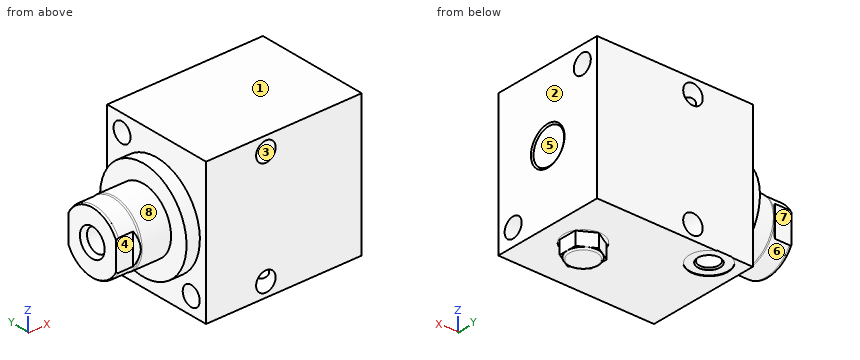
from build123d import *

# Parameters (mm, degrees)
SKETCH1_W            = 63.5
SKETCH1_H            = 50.8
EXTRUDE1_DEPTH       = 69.723
LPATTERN1_COUNT      = 2
LPATTERN1_PITCH      = 41.148
LPATTERN1_COUNT_DIR2 = 2
LPATTERN1_PITCH_DIR2 = 17.4498
SKETCH5_R            = 22.225
EXTRUDE2_DEPTH       = 5.969
SKETCH6_W            = 14.2748
SKETCH6_H            = 22.86
CUT_EXTRUDE4_DEPTH   = 30.48
HOLE1_D              = 8.738
HOLE1_DEPTH          = 69.723
HOLE2_D              = 8.738
HOLE2_DEPTH          = 50.8
EXTRUDE3_DEPTH       = 6.78
SKETCH21_R           = 7.874
EXTRUDE4_DEPTH       = 2.54


with BuildPart() as part:
    # Sketch1 → Extrude1 (new body)
    with BuildSketch(Plane(origin=(0, 0, 0), x_dir=(0, 0, -1), z_dir=(1, 0, 0))):
        Rectangle(SKETCH1_W, SKETCH1_H)
    extrude(amount=EXTRUDE1_DEPTH)

    # S2D0002 → Cut-Revolve1 (revolve, cut)
    with BuildSketch(Plane(origin=(0, 17.4498, 0), x_dir=(-1, 0, 0), z_dir=(0, 1, 0)), mode=Mode.PRIVATE) as cut_revolve1_sk:
        Polygon((-17.7165, -31.496), (-21.336, -31.496), (-21.336, -31.75), (-12.7, -31.75), (-12.7, -18.034), (-17.1196, -18.034), (-17.1196, -30.8737), (-17.7165, -31.4706), align=None)
    cut_revolve1 = revolve(cut_revolve1_sk.sketch.rotate(Axis((12.7, 17.4498, -19.13842003), (0, 0, 1)), 180), axis=Axis((12.7, 17.4498, -19.13842003), (0, 0, 1)), mode=Mode.SUBTRACT)  # turned: the seam where the file's is

    # LPattern1: Cut-Revolve1 2 × 2, 2 skipped
    with Locations(*[(i * LPATTERN1_PITCH, -j * LPATTERN1_PITCH_DIR2, 0) for i in range(LPATTERN1_COUNT) for j in range(LPATTERN1_COUNT_DIR2) if (i, j) not in ((0, 0), (0, 1), (1, 0))]):
        add(cut_revolve1, mode=Mode.SUBTRACT)

    # Sketch5 → Extrude2 (add)
    with BuildSketch(Plane.ZY):
        Circle(SKETCH5_R)
    extrude(amount=EXTRUDE2_DEPTH)

    # Sketch6 → Revolve1 (revolve)
    with BuildSketch(Plane(origin=(0, 0, 0), x_dir=(0, 0, 1), z_dir=(0, -1, 0)), mode=Mode.PRIVATE) as revolve1_sk:
        with Locations((-7.1374, 17.399)):
            Rectangle(SKETCH6_W, SKETCH6_H)
    revolve(revolve1_sk.sketch.rotate(Axis((5.754582971, 0, 0), (-1, 0, 0)), 180), axis=Axis((5.754582971, 0, 0), (-1, 0, 0)))  # turned: the seam where the file's is

    # S2D0001 → Cut-Revolve4 (revolve, cut)
    with BuildSketch(Plane(origin=(-18.511260017, 3.2639, 0), x_dir=(0, 1, 0), z_dir=(0, 0, 1)), mode=Mode.PRIVATE) as cut_revolve4_sk:
        Polygon((1.8669, 8.206023638), (1.8669, -6.522460017), (-3.2639, -6.522460017), (-3.2639, 10.317739983), (3.0861, 10.317739983), align=None)
    revolve(cut_revolve4_sk.sketch.rotate(Axis((0, 0, 0), (-1, 0, 0)), 90), axis=Axis((0, 0, 0), (-1, 0, 0)), mode=Mode.SUBTRACT)  # turned: the seam where the file's is

    # Sketch8 → Cut-Revolve5 (revolve, cut)
    with BuildSketch(Plane(origin=(0, 0, 0), x_dir=(0, 0, -1), z_dir=(0, 1, 0)), mode=Mode.PRIVATE) as cut_revolve5_sk:
        with BuildLine():
            Line((-14.2748, 18.923), (-14.097, 19.685))
            Line((-14.097, 19.685), (-14.097, 27.813))
            ThreePointArc((-14.097, 27.813), (-13.996678675, 28.356796865), (-13.708922533, 28.829))
            Line((-13.708922533, 28.829), (-14.2748, 28.829))
            Line((-14.2748, 28.829), (-14.2748, 18.923))
        make_face()
    revolve(cut_revolve5_sk.sketch.rotate(Axis((-12.65936, 0, 0), (-1, 0, 0)), 180), axis=Axis((-12.65936, 0, 0), (-1, 0, 0)), mode=Mode.SUBTRACT)  # turned: the seam where the file's is

    # Sketch12 → Cut-Extrude4 (cut, symmetric)
    with BuildSketch(Plane(origin=(0, 0, 0), x_dir=(0, -1, 0), z_dir=(0, 0, -1))):
        Polygon((12.319, 28.829), (12.319, 21.2598), (14.2748, 19.304), (14.2748, 28.829), align=None)
        Polygon((-12.319, 28.829), (-12.319, 21.2598), (-14.2748, 19.304), (-14.2748, 28.829), align=None)
    extrude(amount=CUT_EXTRUDE4_DEPTH, both=True, mode=Mode.SUBTRACT)

    # Hole1
    with Locations(Plane.ZY):
        with Locations((-24.13, -17.78), (24.13, 17.78)):
            Hole(HOLE1_D / 2, depth=HOLE1_DEPTH)

    # Hole2
    with Locations(Plane(origin=(0, 25.4, 0), x_dir=(-1, 0, 0), z_dir=(0, 1, 0))):
        with Locations((-26.797, -25.4), (-26.797, 25.4)):
            Hole(HOLE2_D / 2, depth=HOLE2_DEPTH)

    # Sketch18 → Extrude3 (add)
    with BuildSketch(Plane(origin=(0, 0, -31.496), x_dir=(-1, 0, 0), z_dir=(0, 0, -1))):
        Polygon((-46.863, 4.03279163), (-53.848, 8.065583261), (-60.833, 4.03279163), (-60.833, -4.03279163), (-53.848, -8.065583261), (-46.863, -4.03279163), align=None)
    extrude(amount=EXTRUDE3_DEPTH)

    # Sketch19 → Cut-Revolve6 (revolve, cut)
    with BuildSketch(Plane(origin=(0, 0, 0), x_dir=(-1, 0, 0), z_dir=(0, 1, 0)), mode=Mode.PRIVATE) as cut_revolve6_sk:
        with BuildLine():
            Line((-60.071, -38.276), (-60.071, -40.689))
            Line((-60.071, -40.689), (-63.246, -40.689))
            Line((-63.246, -40.689), (-63.246, -37.514))
            Line((-63.246, -37.514), (-60.833, -37.514))
            ThreePointArc((-60.833, -37.514), (-60.609815367, -38.052815367), (-60.071, -38.276))
        make_face()
    revolve(cut_revolve6_sk.sketch.rotate(Axis((53.848, 0, -18.51025594), (0, 0, -1)), 180), axis=Axis((53.848, 0, -18.51025594), (0, 0, -1)), mode=Mode.SUBTRACT)  # turned: the seam where the file's is

    # Sketch20 → Cut-Revolve7 (revolve, cut)
    with BuildSketch(Plane(origin=(0, 0, 0), x_dir=(1, 0, 0), z_dir=(0, 1, 0)), mode=Mode.PRIVATE) as cut_revolve7_sk:
        Polygon((69.723, 8.636), (66.675, 8.636), (66.675, 5.0165), (66.6496, 5.0165), (66.0527, 4.4196), (56.1086, 4.4196), (56.1086, 0), (69.723, 0), align=None)
    revolve(cut_revolve7_sk.sketch.rotate(Axis((0, 0, 0), (1, 0, 0)), 180), axis=Axis((0, 0, 0), (1, 0, 0)), mode=Mode.SUBTRACT)  # turned: the seam where the file's is

    # Sketch21 → Extrude4 (add)
    with BuildSketch(Plane(origin=(66.675, 0, 0), x_dir=(0, 0, -1), z_dir=(1, 0, 0))):
        Circle(SKETCH21_R)
    extrude(amount=EXTRUDE4_DEPTH)


solid = part.part
Could you check a few things on this model? Use its own coordinates, in mm. Face numbers are marked on the shaded views. A direction names the side the tool comes from. Round coordinates to 2 decimals unless told otherwise and drop trailing zeros. Order: outer loops, then holes, each group sorted by start corner. A loop starts at its lowest first (then second) coordinate and runs counter-clockwise, first axis right, second up.
(1) I'm going to push flat-ended pins straight in: pin 1 (3 mm diameter, centred on y = 0, z = 1, fed in from -X); pin 2 (1.5 mm diameter, centred on y = -2, z = -21, fed in from -X); pin 3 (1.6 mm diameter, centred on x = 55, y = -7, fed in from -Z). Where does each tip first touch, or does it pass through?
Response values:
pin 1: stops at x = -11.99
pin 2: stops at x = -5.97
pin 3: stops at z = -38.27
(2) Imagine slicing it at C-C (x = 28.5). Write out the boundary of the cut face in (y, z).
Response values:
outline: (-25.4, -31.75) - (25.4, -31.75) - (25.4, -29.42) - (-25.4, -29.42) - close; (-25.4, -21.38) - (-21.17, -21.38) arc R4.37 cw to (-14.39, -21.38) - (25.4, -21.38) - (25.4, 21.38) - (21.17, 21.38) arc R4.37 cw to (14.39, 21.38) - (-25.4, 21.38) - close; (-25.4, 29.42) - (25.4, 29.42) - (25.4, 31.75) - (-25.4, 31.75) - close
(3) Imagine slicing it at D-D (z = -34). Write out the boundary of the cut face in (x, y).
Response values:
outline: (46.86, -4.03) - (53.85, -8.07) - (60.83, -4.03) - (60.83, 4.03) - (53.85, 8.07) - (46.86, 4.03) - close
(4) Which directions (+Z, -Z, +X, -X, +Y, -Y) give clear straight access to the entire face, cutting with the end or side of a thin tool? Please do the marked faces 4, 5, 6, 7 and 8.
Response values:
face 4: +Z, -Z, -X, -Y
face 5: +X
face 6: -Z, -X
face 7: +Z, -Z, -X, +Y
face 8: -X
(5) Imagine slicing it at A-A (x = 39.5). Write out the boundary of the cut face in (y, z), plus the area to 3 significant figures.
Response values:
outline: (-25.4, -31.75) - (25.4, -31.75) - (25.4, 31.75) - (-25.4, 31.75) - close; hole circle Ø8.74 at (-17.78, -24.13); hole circle Ø8.74 at (17.78, 24.13)
area: 3,110 mm2
(6) If we mould it in two halves opening along Z, with no side actions, what happens to the marked faces 1, 2 and 3? For each: released by +Z, released by -Z, zero draft, split by the parting line, or undercut.
Response values:
face 1: released by +Z
face 2: zero draft
face 3: undercut
(7) Imagine slicing it at B-B (z = -24.13). Write out the boundary of the cut face in (x, y), plus the area to 3 significant figures.
Response values:
outline: (0, -25.4) - (22.62, -25.4) - (22.62, -22.15) - (0, -22.15) - close; (0, -13.41) - (22.62, -13.41) - (22.62, 25.4) - (0, 25.4) - close; (30.98, -25.4) - (69.72, -25.4) - (69.72, -22.15) - (30.98, -22.15) - close; (30.98, -13.41) - (69.72, -13.41) - (69.72, 25.4) - (30.98, 25.4) - close; hole circle Ø8.84 at (12.7, 17.45); hole circle Ø8.84 at (53.85, 0)
area: 2,460 mm2
(8) Please list where these lines run through material, in increasing order: line 1 along Y through (x, z) = (-15.75, 0); line 2 along X through (y, z) = (19, -22.5); line 3 along Y through (x, z) = (57.5, -27.5).
Response values:
line 1: y = -14.27 to -5.13, 5.13 to 14.27
line 2: x = 0 to 8.56, 16.84 to 23.53, 30.06 to 69.72
line 3: y = -25.4 to -20.56, -15 to -2.49, 2.49 to 25.4
